Design review of the part built by this model. Coordinates are the model's own, in mm. A direction names the side the tool comes from. Coordinates: 2 decimals unless noted, no trailing zeros. Loops run counter-clockwise (first coordinate to the right, second up) from the corner with the lowest first, then second, coordinate; pieces in that order, holes last. Notation, with made-up numbers: (68.5, 10.5) - (82.5, 10.5) arc R33 ccw to (82.5, 46.5) - close; hole circle Ø6 at (63, -39). An arc over 180 degrees is marked (long way). Use one line per item in the form item = value. Start each with the question number.
(1) Add section D-D (z = -50.5). State the section outline as (x, y) points.
(2) The part is to be moulded in two halves that separate along Y. For faces 1 (the face through (1, 35, -9.5)), 2 (the face through (6.44, 28.24, -42.07)), 3 (the face through (6, 88, -55)), say which applies: pulls with the +Y half, pulls with the -Y half, needs draft (parallel to the pull), parting line crosses it, or undercut.
(3) Tool access review of faces 4 (the face through (15, 88, -10)), 5 (the face through (1.479, 67.886, -50.184)), 6 (the face through (10, 85, -17)), 7 (the face through (14, 88, -45)), 8 (the face through (15.711, 92.538, -26.948)): name each direction out of +Z, -Z, +X, -X, +Y, -Y from which nothing blocks a thin tool from reaching the whole face with its end or side.
(4) Clearance check with flat-ended pins moving along their axes: pin 1 Ø7.5 at (y, z) = (72.5, -51) entering from -X; pin 2 Ø3.5 at (x, y) = (1, 37) entering from +Z; pin 3 Ø1.5 at (x, y) = (1, 73) entering from -Z. State where each tip first meets the part, or that it passes through.
(5) For L1, parallel to Y at x = 15.5, z = -28; L2, parallel to X at y = 16, z = -42.5; L3, parallel to Z at x = 6.5, y = 6.75, list the stretches that pass through material, from the lowest coordinate up.
(6) Add section B-B (y = 51.5). State the section outline as (x, z) points, plus the area to 3 significant figures.
(7) Add section C-C (y = 21). State the section outline as (x, z) points.
```python
from build123d import *

# Parameters (mm, degrees)
BOSS_EXTRUDE1_DEPTH   = 180
SKETCH3_R             = 11.2
CUT_EXTRUDE1_DEPTH    = 17.5
SKETCH11_W            = 1.6
SKETCH11_H            = 1.8
LPATTERN1_COUNT       = 2
LPATTERN1_PITCH       = 60
M6_TAPPED_HOLE1_D     = 5
M6_TAPPED_HOLE1_DEPTH = 27
M6_TAPPED_HOLE1_TIP   = 1.502151548
CUT_EXTRUDE2_DEPTH    = 3
FILLET1_R             = 1
SKETCH16_R            = 16.086182712
BOSS_EXTRUDE2_DEPTH   = 16.5


with BuildPart() as part:
    # Sketch1 → Boss-Extrude1 (new body)
    with BuildSketch(Plane(origin=(0, 0, 0), x_dir=(1, 0, 0), z_dir=(0, 1, 0))):
        Polygon((0, 0), (0, 55), (12.5, 55), (12.5, 45), (16.5, 45), (16.5, 10), (12.5, 10), (12.5, 0), align=None)
    extrude(amount=BOSS_EXTRUDE1_DEPTH)

    # Sketch3 → Cut-Extrude1 (cut, through all)
    with BuildSketch(Plane(origin=(16.5, 0, 0), x_dir=(0, 0, -1), z_dir=(1, 0, 0))):
        with Locations((27.5, 80)):
            Circle(SKETCH3_R)
    cut_extrude1 = extrude(amount=-CUT_EXTRUDE1_DEPTH, mode=Mode.SUBTRACT)

    # Sketch11 → Cut-Revolve1 (revolve, cut)
    with BuildSketch(Plane.XY.offset(-27.5)):
        with BuildLine():
            Line((10, 69.15), (12.5, 69.15))
            Line((12.5, 69.15), (12.5, 67.55))
            ThreePointArc((12.5, 67.55), (12.441421356, 67.408578644), (12.3, 67.35))
            Line((12.3, 67.35), (10.2, 67.35))
            ThreePointArc((10.2, 67.35), (10.058578644, 67.408578644), (10, 67.55))
            Line((10, 67.55), (10, 69.15))
        make_face()
        with Locations((15.7, 66.55)):
            Rectangle(SKETCH11_W, SKETCH11_H)
    cut_revolve1 = revolve(axis=Axis((16.5, 80, -27.5), (-1, 0, 0)), mode=Mode.SUBTRACT)

    # LPattern1: Cut-Extrude1, Cut-Revolve1 ×2
    with Locations(*[(0, i * LPATTERN1_PITCH, 0) for i in range(1, LPATTERN1_COUNT)]):
        add(cut_extrude1, mode=Mode.SUBTRACT)
        add(cut_revolve1, mode=Mode.SUBTRACT)

    # M6 Tapped Hole1
    with Locations(Plane.XZ):
        with Locations((6.5, -12.5), (6.5, -42.5)):
            Hole(M6_TAPPED_HOLE1_D / 2, depth=M6_TAPPED_HOLE1_DEPTH)
            with Locations((0, 0, -(M6_TAPPED_HOLE1_DEPTH + M6_TAPPED_HOLE1_TIP / 2))):  # 118° drill point
                Cone(0, M6_TAPPED_HOLE1_D / 2, M6_TAPPED_HOLE1_TIP, mode=Mode.SUBTRACT)

    # Sketch15 → Cut-Extrude2 (cut)
    with BuildSketch(Plane.ZY):
        Polygon((-55, 144.75), (-45.5, 146.75), (-45.5, 133.25), (-55, 135.25), align=None)
        Polygon((-55, 78.4), (-45.5, 80.4), (-45.5, 66.9), (-55, 68.9), align=None)
        Polygon((0, 39.2), (-9.5, 41.2), (-9.5, 27.7), (0, 29.7), align=None)
    extrude(amount=-CUT_EXTRUDE2_DEPTH, mode=Mode.SUBTRACT)

    # Fillet1
    fillet1_edges = [part.edges().sort_by_distance(p)[0] for p in [
        (14.5, 180, -10),
        (16.5, 180, -27.5),
        (0, 109.6, 0),
        (0, 162.375, -55),
        (12.5, 90, -55),
        (12.5, 90, 0),
        (14.5, 180, -45),
        (12.5, 180, -50),
        (6.25, 180, -55),
        (0, 180, -27.5),
        (6.25, 180, 0),
        (12.5, 180, -5),
        (0, 106.825, -55),
        (0, 34.45, -55),
        (0, 14.85, 0),
    ]]
    fillet(fillet1_edges, radius=FILLET1_R)

    # Sketch16 → Boss-Extrude2 (add)
    with BuildSketch(Plane(origin=(16.5, 0, 0), x_dir=(0, 0, -1), z_dir=(1, 0, 0))):
        with Locations((27.5, 140)):
            Circle(SKETCH16_R)
    extrude(amount=-BOSS_EXTRUDE2_DEPTH)


solid = part.part
```
Computed values:
q1.outline = (0, 0) - (12.5, 0) - (12.5, 179) arc R1 ccw to (11.5, 180) - (1, 180) arc R1 ccw to (0, 179) - (0, 145.7) - (3, 145.7) - (3, 134.3) - (0, 134.3) - (0, 79.35) - (3, 79.35) - (3, 67.95) - (0, 67.95) - close
q2.face_1 = undercut
q2.face_2 = pulls with the -Y half
q2.face_3 = needs draft
q3.face_4 = +Z, +X, +Y, -Y
q3.face_5 = -X
q3.face_6 = none
q3.face_7 = -Z, +X, +Y, -Y
q3.face_8 = +X
q4.pin_1 = 3
q4.pin_2 = -9.5
q4.pin_3 = -45.5
q5.L1 = 0 to 65.66, 67.46 to 68.81, 91.19 to 92.54, 94.34 to 180
q5.L2 = 0 to 4, 9 to 16.5
q5.L3 = -55 to -45, -40 to -15, -10 to 0
q6.outline = (0, -54) arc R1 ccw to (1, -55) - (11.5, -55) arc R1 ccw to (12.5, -54) - (12.5, -45) - (16.5, -45) - (16.5, -10) - (12.5, -10) - (12.5, -1) arc R1 ccw to (11.5, 0) - (1, 0) arc R1 ccw to (0, -1) - close
q6.area = 827 mm^2
q7.outline = (0, -54) arc R1 ccw to (1, -55) - (11.5, -55) arc R1 ccw to (12.5, -54) - (12.5, -45) - (16.5, -45) - (16.5, -10) - (12.5, -10) - (12.5, -1) arc R1 ccw to (11.5, 0) - (1, 0) arc R1 ccw to (0, -1) - close; hole circle Ø5 at (6.5, -42.5); hole circle Ø5 at (6.5, -12.5)
